Build history of the part. All positions in model axes, mm. A direction names the side the tool comes from. Coordinates: 2 decimals unless noted, no trailing zeros. Write each loop counter-clockwise with the first axis right and the second up, starting at its lowest first coordinate (ties: lowest second). Pieces come first, ordered by that corner, then holes.
```python
from build123d import *

# Parameters (mm, degrees)
SKETCH_1_R          = 2.5
EXTRUDE_1_DEPTH     = 1.6
SKETCH_2_R          = 1.5
EXTRUDE_2_DEPTH     = 30
CUT_EXTRUDE_1_DEPTH = 1


with BuildPart() as part:
    # 草图1 → 凸台-拉伸1 (new body)
    with BuildSketch(Plane(origin=(0, 0, 0), x_dir=(1, 0, 0), z_dir=(0, 1, 0))):
        Circle(SKETCH_1_R)
    extrude(amount=EXTRUDE_1_DEPTH)

    # 草图2 → 凸台-拉伸2 (add)
    with BuildSketch(Plane(origin=(0, 1.6, 0), x_dir=(1, 0, 0), z_dir=(0, 1, 0))):
        Circle(SKETCH_2_R)
    extrude(amount=EXTRUDE_2_DEPTH)

    # 草图3 → 切除-拉伸1 (cut)
    with BuildSketch(Plane.XZ):
        with BuildLine():
            Line((-0.5, 1), (-0.5, 1.75))
            Line((-0.5, 1.75), (0.5, 1.75))
            Line((0.5, 1.75), (0.5, 1))
            ThreePointArc((0.5, 1), (0.646446609, 0.646446609), (1, 0.5))
            Line((1, 0.5), (1.75, 0.5))
            Line((1.75, 0.5), (1.75, -0.5))
            Line((1.75, -0.5), (1, -0.5))
            ThreePointArc((1, -0.5), (0.646446609, -0.646446609), (0.5, -1))
            Line((0.5, -1), (0.5, -1.75))
            Line((0.5, -1.75), (-0.5, -1.75))
            Line((-0.5, -1.75), (-0.5, -1))
            ThreePointArc((-0.5, -1), (-0.646446609, -0.646446609), (-1, -0.5))
            Line((-1, -0.5), (-1.75, -0.5))
            Line((-1.75, -0.5), (-1.75, 0.5))
            Line((-1.75, 0.5), (-1, 0.5))
            ThreePointArc((-1, 0.5), (-0.646446609, 0.646446609), (-0.5, 1))
        make_face()
    extrude(amount=-CUT_EXTRUDE_1_DEPTH, mode=Mode.SUBTRACT)


solid = part.part
```
1. Mould opens along Z. For faces 1 (the face through (-0.54, 0.79, 2.44)), 2 (the face through (0, 1, 0)), 3 (the face through (0, 31.6, 0)) say: +Z half, -Z half, draft (parallel to the pull), parting line (faces both ways), or undercut.
Computed values:
face 1: parting line
face 2: undercut
face 3: draft
2. Probe line 1 along Y through (x, z) = (1.4, 1.7); line 2 along X through (y, z) = (29, 0.05). List the from-to ranges inside material, lowest first.
Computed values:
line 1: y = 0 to 1.6
line 2: x = -1.5 to 1.5
3. Flat gauge pins, fed straight in: pin 1 (1 mm diameter, centred on x = 0.5, y = 5, fed in from -Z); pin 2 (0.8 mm diameter, centred on y = 0.5, z = 1.5, fed in from -X) (3 decimals); pin 3 (2 mm diameter, centred on x = 1.5, y = 22, fed in from -Z). Where does each tip first touch, or does it go through?
Computed values:
pin 1: stops at z = -1.5
pin 2: stops at x = -2.245
pin 3: stops at z = -1.41
4. Saw through at C-C on y = 26. List the corners of the cut face in (x, z).
Computed values:
outline: circle Ø3 at (0, 0)
5. 3-axis set-ups, long thin cutter, end or side, ignore diameter. For faces 4 (the face through (1, 0, 1)), 5 (the face through (0, 0.5, 1.75)), 6 (the face through (-1.5, 16.39, -0.07)): which of +Z, -Z, +X, -X, +Y, -Y reach the whole face in a straight line?
Computed values:
face 4: +Z, -Z, +X, -X, -Y
face 5: -Y
face 6: +Y
6. Saw through at D-D on x = 2.05. List the corners of the cut face in (y, z), plus the area to 3 significant figures.
Computed values:
outline: (0, -1.43) - (1.6, -1.43) - (1.6, 1.43) - (0, 1.43) - close
area: 4.58 mm2
7. Saw through at A-A on z = 0. List the corners of the cut face in (x, y), plus the area to 3 significant figures.
Computed values:
outline: (-2.5, 0) - (-1.75, 0) - (-1.75, 1) - (1.75, 1) - (1.75, 0) - (2.5, 0) - (2.5, 1.6) - (1.5, 1.6) - (1.5, 31.6) - (-1.5, 31.6) - (-1.5, 1.6) - (-2.5, 1.6) - close
area: 94.5 mm2
8. Saw through at B-B on x = 0. List the corners of the cut face in (y, z).
Computed values:
outline: (0, -2.5) - (1.6, -2.5) - (1.6, -1.5) - (31.6, -1.5) - (31.6, 1.5) - (1.6, 1.5) - (1.6, 2.5) - (0, 2.5) - (0, 1.75) - (1, 1.75) - (1, -1.75) - (0, -1.75) - close
